Design review of the part built by this model. Coordinates are the model's own, in mm. Round coordinates to 2 decimals unless told otherwise and drop trailing zeros. Loops run counter-clockwise (first coordinate to the right, second up) from the corner with the lowest first, then second, coordinate; pieces in that order, holes last. Notation, with made-up numbers: (-17, 29) - (18, 29) arc R19 cw to (18, 44) - close; hole circle Ø7 at (1.5, 44). An arc over 180 degrees is marked (long way). Return JSON: item names as keys, results as strings. Group by question number.
(1) We need section B-B, the plane x = 26.67. Write out the cut boundary in (y, z), and give its area (3 significant figures).
(2) We need section D-D, the plane x = 0. Write out the cut boundary in (y, z).
(3) Wall thickness on L1, parallel to X at y = 1.35, z = 33; L2, parallel to Z at x = -49.5, y = 1.15; L3, parallel to X at y = 1.35, z = -3: over which ranges is each line inside the solid? List them lowest first. Write a range as [from, to].
(4) Clearance check with flat-ended pins moving along their axes: pin 1 (2 mm diameter, centred on y = 2.5, z = -7.5, fed in from +X); pin 2 (2 mm diameter, centred on x = -27, y = 4, fed in from +Z). State where each tip first meets the part, or that it passes through.
(5) We need section A-A, the plane z = -33.02. Write out the cut boundary in (x, y), and give its area (3 significant figures).
(6) We need section C-C, the plane y = 1.25. Give the number of separate pieces and of enclosed holes in the cut face, and give its area (3 significant figures).
from build123d import *

# Parameters (mm, degrees)
SKETCH1_R           = 1.5875
BOSS_EXTRUDE1_DEPTH = 4.7625
SKETCH11_R          = 2.54
SKETCH11_R_2        = 1.143
CUT_EXTRUDE1_DEPTH  = 90.928757393


with BuildPart() as part:
    # Sketch1 → Boss-Extrude1 (new body)
    with BuildSketch(Plane(origin=(0, 0, 0), x_dir=(1, 0, 0), z_dir=(0, 1, 0))):
        with BuildLine():
            ThreePointArc((-48.380952381, 63.267486058), (-59.780256121, 59.780256121), (-63.267486058, 48.380952381))
            ThreePointArc((-63.267486058, 48.380952381), (-58.617207227, 0), (-63.267486058, -48.380952381))
            ThreePointArc((-63.267486058, -48.380952381), (-59.780256121, -59.780256121), (-48.380952381, -63.267486058))
            ThreePointArc((-48.380952381, -63.267486058), (0, -58.617207227), (48.380952381, -63.267486058))
            ThreePointArc((48.380952381, -63.267486058), (59.780256121, -59.780256121), (63.267486058, -48.380952381))
            ThreePointArc((63.267486058, -48.380952381), (58.617207227, 0), (63.267486058, 48.380952381))
            ThreePointArc((63.267486058, 48.380952381), (59.780256121, 59.780256121), (48.380952381, 63.267486058))
            ThreePointArc((48.380952381, 63.267486058), (0, 58.617207227), (-48.380952381, 63.267486058))
        make_face()
        with Locations(Location((-26.67, 33.02, 0), (0, 0, 90))):
            Circle(SKETCH1_R, mode=Mode.SUBTRACT)
        with Locations(Location((26.67, 33.02, 0), (0, 0, 90))):
            Circle(SKETCH1_R, mode=Mode.SUBTRACT)
        with Locations(Location((-26.67, -33.02, 0), (0, 0, 90))):
            Circle(SKETCH1_R, mode=Mode.SUBTRACT)
        with Locations(Location((26.67, -33.02, 0), (0, 0, 90))):
            Circle(SKETCH1_R, mode=Mode.SUBTRACT)
    extrude(amount=BOSS_EXTRUDE1_DEPTH)

    # Sketch11 → Cut-Extrude1 (cut, through all)
    with BuildSketch(Plane(origin=(0, 4.7625, 0), x_dir=(1, 0, 0), z_dir=(0, 1, 0))):
        with Locations(Location((-50.8, 50.8, 0), (0, 0, 270))):
            Circle(SKETCH11_R)
        with Locations(Location((-42.418, 50.8, 0), (0, 0, 270))):
            Circle(SKETCH11_R_2)
        with Locations(Location((-50.8, 42.418, 0), (0, 0, 270))):
            Circle(SKETCH11_R_2)
        with Locations(Location((-59.182, 50.8, 0), (0, 0, 270))):
            Circle(SKETCH11_R_2)
        with Locations(Location((-50.8, 59.182, 0), (0, 0, 270))):
            Circle(SKETCH11_R_2)
        with Locations(Location((50.8, 50.8, 0), (0, 0, 270))):
            Circle(SKETCH11_R)
        with Locations(Location((59.182, 50.8, 0), (0, 0, 270))):
            Circle(SKETCH11_R_2)
        with Locations(Location((50.8, 42.418, 0), (0, 0, 270))):
            Circle(SKETCH11_R_2)
        with Locations(Location((42.418, 50.8, 0), (0, 0, 270))):
            Circle(SKETCH11_R_2)
        with Locations(Location((50.8, 59.182, 0), (0, 0, 270))):
            Circle(SKETCH11_R_2)
        with Locations(Location((50.8, -50.8, 0), (0, 0, 270))):
            Circle(SKETCH11_R)
        with Locations(Location((59.182, -50.8, 0), (0, 0, 270))):
            Circle(SKETCH11_R_2)
        with Locations(Location((50.8, -59.182, 0), (0, 0, 270))):
            Circle(SKETCH11_R_2)
        with Locations(Location((42.418, -50.8, 0), (0, 0, 270))):
            Circle(SKETCH11_R_2)
        with Locations(Location((50.8, -42.418, 0), (0, 0, 270))):
            Circle(SKETCH11_R_2)
        with Locations(Location((-50.8, -50.8, 0), (0, 0, 270))):
            Circle(SKETCH11_R)
        with Locations(Location((-42.418, -50.8, 0), (0, 0, 270))):
            Circle(SKETCH11_R_2)
        with Locations(Location((-50.8, -59.182, 0), (0, 0, 270))):
            Circle(SKETCH11_R_2)
        with Locations(Location((-59.182, -50.8, 0), (0, 0, 270))):
            Circle(SKETCH11_R_2)
        with Locations(Location((-50.8, -42.418, 0), (0, 0, 270))):
            Circle(SKETCH11_R_2)
    extrude(amount=-CUT_EXTRUDE1_DEPTH, mode=Mode.SUBTRACT)


solid = part.part
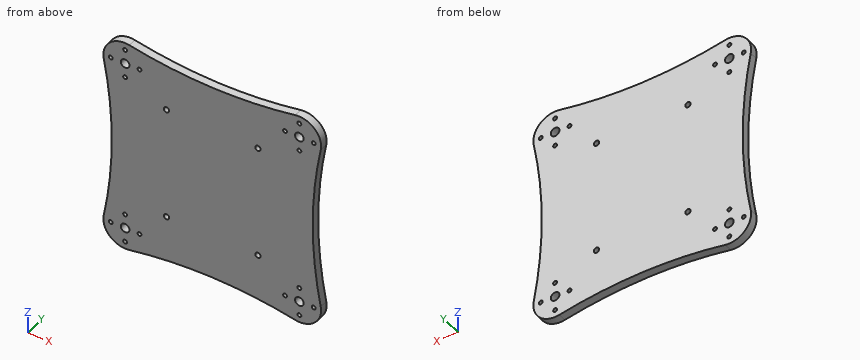
Solutions:
{
 "1": {"outline": "(0, -60.02) - (4.76, -60.02) - (4.76, -34.61) - (0, -34.61) - close; (0, -31.43) - (4.76, -31.43) - (4.76, 31.43) - (0, 31.43) - close; (0, 34.61) - (4.76, 34.61) - (4.76, 60.02) - (0, 60.02) - close", "area": "541 mm^2"},
 "2": {"outline": "(0, -58.62) - (4.76, -58.62) - (4.76, 58.62) - (0, 58.62) - close"},
 "3": {"L1": "[-60.77, -28.26], [-25.08, 25.08], [28.26, 60.77]", "L2": "[-63.43, -52.98], [-48.62, 48.62], [52.98, 63.43]", "L3": "[-58.63, 58.63]"},
 "4": {"pin 1": "x = 58.76", "pin 2": "z = 60.17"},
 "5": {"outline": "(-60.77, 0) - (-28.26, 0) - (-28.26, 4.76) - (-60.77, 4.76) - close; (-25.08, 0) - (25.08, 0) - (25.08, 4.76) - (-25.08, 4.76) - close; (28.26, 0) - (60.77, 0) - (60.77, 4.76) - (28.26, 4.76) - close", "area": "549 mm^2"},
 "6": {"separate pieces": "1", "enclosed holes": "24", "area": "14,500 mm^2"}
}
